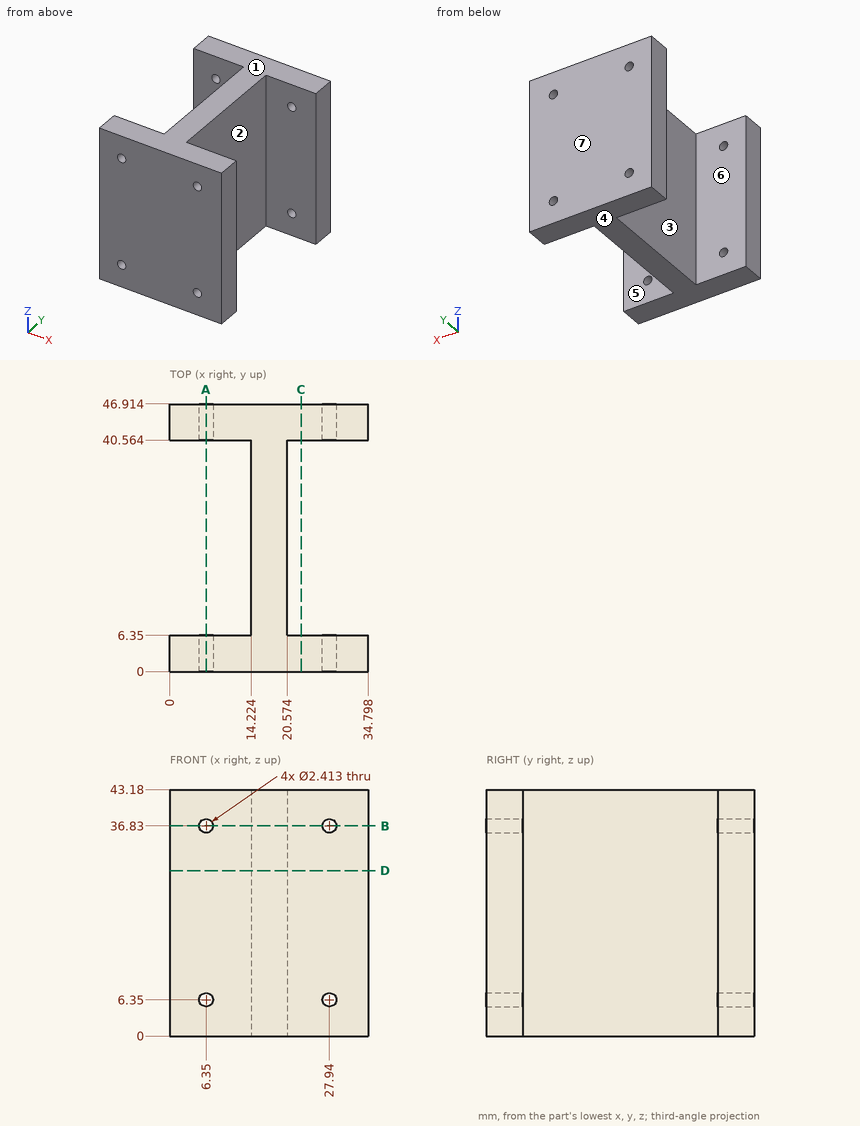
The drawing under review shows one solid part. Ordinate dimensions are in mm from its lowest x, y, z. A direction names the side the tool comes from. Round coordinates to 2 decimals unless told otherwise and drop trailing zeros. Write each loop counter-clockwise with the first axis right and the second up, starting at its lowest first coordinate (ties: lowest second). Pieces come first, ordered by that corner, then holes.
(1) Wall thickness on L1, parallel to Z at x = 6.35, y = 42.25; L2, parallel to Y at x = 10, z = 16; L3, parallel to X at y = 44, z = 6 (1 decimal): over which ranges is each line inside the solid? List them lowest first.
(2) Insertion check: pin 1 (10.5 mm diameter, centred on y = 23, z = 11.5, fed in from -X); pin 2 (4 mm diameter, centred on y = 33, z = 19, fed in from +X). Each pin has a flat end and moves straight along its axis. Give the tip position at first contact, or say it passes through.
(3) We need section C-C on x = 23. Give the boundary of the cut face in (y, z), and give its area (3 significant figures).
(4) Machinability: for the marked faces 1, 2 and 3, which of the approach directions +Z, -Z, +X, -X, +Y, -Y give a long, thin tool a straight path to every point of the face, cutting with its end or side? Answer none if there is none.
(5) We need section B-B on z = 36.83. Give the boundary of the cut face in (x, y).
(6) We need section A-A on x = 6.35. Give the boundary of the cut face in (y, z).
(7) Mouldability with a two-part tool opening along Y and no side actions: class the marked faces 4, 5, 6 and 7 as +Y half, -Y half, draft (parallel to the pull), parting line (faces both ways), or undercut.
(8) We need section D-D on z = 29. Give the boundary of the cut face in (x, y).
Findings below:
1. L1: z = 0 to 5.14, 7.56 to 35.62, 38.04 to 43.18
1. L2: y = 0 to 6.35, 40.56 to 46.91
1. L3: x = 0 to 5.2, 7.5 to 26.8, 29.1 to 34.8
2. pin 1: stops at x = 14.22
2. pin 2: stops at x = 20.57
3. outline: (0, 0) - (6.35, 0) - (6.35, 43.18) - (0, 43.18) - close; (40.56, 0) - (46.91, 0) - (46.91, 43.18) - (40.56, 43.18) - close
3. area: 548 mm2
4. face 1: +Z, +X, -X, +Y, -Y
4. face 2: +Z, -Z, +X
4. face 3: +Z, -Z, -X
5. outline: (0, 0) - (5.14, 0) - (5.14, 6.35) - (0, 6.35) - close; (0, 40.56) - (5.14, 40.56) - (5.14, 46.91) - (0, 46.91) - close; (7.56, 0) - (26.73, 0) - (26.73, 6.35) - (20.57, 6.35) - (20.57, 40.56) - (26.73, 40.56) - (26.73, 46.91) - (7.56, 46.91) - (7.56, 40.56) - (14.22, 40.56) - (14.22, 6.35) - (7.56, 6.35) - close; (29.15, 0) - (34.8, 0) - (34.8, 6.35) - (29.15, 6.35) - close; (29.15, 40.56) - (34.8, 40.56) - (34.8, 46.91) - (29.15, 46.91) - close
6. outline: (0, 0) - (6.35, 0) - (6.35, 5.14) - (0, 5.14) - close; (0, 7.56) - (6.35, 7.56) - (6.35, 35.62) - (0, 35.62) - close; (0, 38.04) - (6.35, 38.04) - (6.35, 43.18) - (0, 43.18) - close; (40.56, 0) - (46.91, 0) - (46.91, 5.14) - (40.56, 5.14) - close; (40.56, 7.56) - (46.91, 7.56) - (46.91, 35.62) - (40.56, 35.62) - close; (40.56, 38.04) - (46.91, 38.04) - (46.91, 43.18) - (40.56, 43.18) - close
7. face 4: draft
7. face 5: undercut
7. face 6: undercut
7. face 7: +Y half
8. outline: (0, 0) - (34.8, 0) - (34.8, 6.35) - (20.57, 6.35) - (20.57, 40.56) - (34.8, 40.56) - (34.8, 46.91) - (0, 46.91) - (0, 40.56) - (14.22, 40.56) - (14.22, 6.35) - (0, 6.35) - close
